from build123d import *

# Parameters (mm, degrees)
SKETCH1_W                         = 101.6
SKETCH1_H                         = 38.1
BASE_FLANGE1_DEPTH                = 3.175
EDGE_FLANGE1_STRIP_W              = 15.748
EDGE_FLANGE1_STRIP_H              = 3.175
EDGE_FLANGE1_STRIP_CUT_DEPTH      = 101.6
EDGE_FLANGE1_DEPTH                = 101.6
F_1_4_CLEARANCE_HOLE1_D           = 6.7564
F_1_4_CLEARANCE_HOLE1_ON_FACE_2_D = 6.7564


# Sheet-metal steps are written as plain solids
with BuildPart() as part:
    # Sketch1 → Base-Flange1 (new body)
    with BuildSketch(Plane.XY):
        with Locations((50.8, 19.05)):
            Rectangle(SKETCH1_W, SKETCH1_H)
    extrude(amount=-BASE_FLANGE1_DEPTH)

    # Edge-Flange1 strip (across the edge) → Edge-Flange1 strip cut (cut)
    with BuildSketch(Plane(origin=(101.6, 38.1, 0), x_dir=(0, -1, 0), z_dir=(-1, 0, 0))):
        with Locations((-3.175, -1.5875)):
            Rectangle(EDGE_FLANGE1_STRIP_W, EDGE_FLANGE1_STRIP_H)
    extrude(amount=EDGE_FLANGE1_STRIP_CUT_DEPTH, mode=Mode.SUBTRACT)

    # Edge-Flange1 section (across the edge) → Edge-Flange1 (add)
    with BuildSketch(Plane(origin=(101.6, 38.1, 0), x_dir=(0, -1, 0), z_dir=(-1, 0, 0))):
        with BuildLine():
            Line((0, 1.524), (0, 28.575))
            Line((0, 28.575), (3.175, 28.575))
            Line((3.175, 28.575), (3.175, 1.524))
            ThreePointArc((3.175, 1.524), (3.621369265, 0.446369265), (4.699, 0))
            Line((4.699, 0), (4.699, -3.175))
            ThreePointArc((4.699, -3.175), (1.376305235, -1.798694765), (0, 1.524))
        make_face()
    extrude(amount=EDGE_FLANGE1_DEPTH)

    # 1/4 Clearance Hole1 (through all)
    with Locations(Plane(origin=(82.55, 16.7005, 0), x_dir=(1, 0, 0), z_dir=(0, 0, 1))):
        with Locations((0, 0), (-31.75, 0), (-63.5, 0)):
            Hole(F_1_4_CLEARANCE_HOLE1_D / 2)

    # 1/4 Clearance Hole1 on face 2 (through all)
    with Locations(Plane(origin=(82.55, 34.925, 19.05), x_dir=(0, 0, -1), z_dir=(0, -1, 0))):
        with Locations((0, 0), (0, -31.75), (0, -63.5)):
            Hole(F_1_4_CLEARANCE_HOLE1_ON_FACE_2_D / 2)


solid = part.part
CAD build for the part. Positions are in the model's coordinates, mm. A direction names the side the tool comes from. Coordinates: 2 decimals unless noted, no trailing zeros. Write each loop counter-clockwise with the first axis right and the second up, starting at its lowest first coordinate (ties: lowest second). Pieces come first, ordered by that corner, then holes. Notation, with made-up numbers: (38.5, 81.5) - (82.5, 81.5) arc R13 ccw to (82.5, 96.5) - close; hole circle Ø1 at (75, -1). An arc over 180 degrees is marked (long way). Use a Markdown table: item, result. Add a question column.
Item 1: Drill centre lines: L1, parallel to X at y = 37.35, z = 19.05; L2, parallel to X at y = 19, z = -0.5; L3, parallel to Z at x = 96.5, y = 6.5 (3 decimals). Where is each one in solid material? Low to high. Write a range as from..to.
Item 2: Band-saw the part on A-A, the plane x = 19.05. Give the cut face in (y, z) (3 decimals), and give its area (3 significant figures).
Item 3: Mould opens along Y. For faces 1 (the face through (19.782, 13.403, -1.61)), 2 (the face through (52, 38.1, 15)), 3 (the face through (50, 13, 0)) say: pulls with the +Y half, pulls with the -Y half, needs draft (parallel to the pull), parting line crosses it, or undercut.
Item 4: Flat gauge pins, fed straight in: pin 1 (3 mm diameter, centred on x = 29.5, y = 18, fed in from +Z); pin 2 (5 mm diameter, centred on x = 13, z = 12.5, fed in from -Y) (3 decimals). Where does each tip first touch, or does it go through?
Item 5: Band-saw the part on B-B, the plane z = 19.05. Give the cut face in (x, y) (3 decimals), and give its area (3 significant figures).
Item 6: 3-axis set-ups, long thin cutter, end or side, ignore diameter. For faces 4 (the face through (52, 37, 28.575)), 5 (the face through (52, 34.925, 15)): which of +Z, -Z, +X, -X, +Y, -Y reach the whole face in a straight line?
Item 7: Band-saw the part on C-C, the plane y = 12. Give the cut face in (x, z) (3 decimals).
Item 8: Band-saw the part on D-D, the plane z = 24.5. Give the cut face in (x, y) (3 decimals).
Numbers:
| question | item | result |
|---|---|---|
| 1 | L1 | 0..15.67, 22.43..47.42, 54.18..79.17, 85.93..101.6 |
| 1 | L2 | 0..16.58, 21.52..48.33, 53.27..80.08, 85.02..101.6 |
| 1 | L3 | -3.175..0 |
| 2 | outline | (0, -3.175) - (13.322, -3.175) - (13.322, 0) - (0, 0) - close; (20.079, -3.175) - (33.401, -3.175) arc R4.699 ccw to (38.1, 1.524) - (38.1, 15.672) - (34.925, 15.672) - (34.925, 1.524) arc R1.524 cw to (33.401, 0) - (20.079, 0) - close; (34.925, 22.428) - (38.1, 22.428) - (38.1, 28.575) - (34.925, 28.575) - close |
| 2 | area | 165 mm2 |
| 3 | face 1 | undercut |
| 3 | face 2 | pulls with the +Y half |
| 3 | face 3 | needs draft |
| 4 | pin 1 | z = 0 |
| 4 | pin 2 | y = 34.925 |
| 5 | outline | (0, 34.925) - (15.672, 34.925) - (15.672, 38.1) - (0, 38.1) - close; (22.428, 34.925) - (47.422, 34.925) - (47.422, 38.1) - (22.428, 38.1) - close; (54.178, 34.925) - (79.172, 34.925) - (79.172, 38.1) - (54.178, 38.1) - close; (85.928, 34.925) - (101.6, 34.925) - (101.6, 38.1) - (85.928, 38.1) - close |
| 5 | area | 258 mm2 |
| 6 | face 4 | +Z, +X, -X, +Y, -Y |
| 6 | face 5 | +Z, +X, -X, -Y |
| 7 | outline | (0, -3.175) - (101.6, -3.175) - (101.6, 0) - (0, 0) - close |
| 8 | outline | (0, 34.925) - (101.6, 34.925) - (101.6, 38.1) - (0, 38.1) - close |
